```python
from build123d import *

# Parameters (mm, degrees)
SKETCH_1_W          = 8
SKETCH_1_H          = 20
EXTRUDE_1_DEPTH     = 10
EXTRUDE_1_2_DEPTH   = 10
SKETCH_2_W          = 39
SKETCH_2_H          = 15
EXTRUDE_2_DEPTH     = 2.5
CHAMFER_1_SIZE      = 1
SKETCH_3_R          = 2
CUT_EXTRUDE_1_DEPTH = 10
CUT_EXTRUDE_3_DEPTH = 10
SKETCH_6_W          = 5
SKETCH_6_H          = 17.5
EXTRUDE_3_DEPTH     = 8
SKETCH_7_W          = 5
SKETCH_7_H          = 17.5
EXTRUDE_4_DEPTH     = 8
EXTRUDE_5_REACH     = 41.825
SKETCH_8_W          = 5
SKETCH_8_H          = 11


with BuildPart() as part:
    # Sketch 1 → Extrude 1 (new body)
    with BuildSketch(Plane.XY):
        with Locations((4, 10)):
            Rectangle(SKETCH_1_W, SKETCH_1_H)
    extrude(amount=EXTRUDE_1_DEPTH)



with BuildPart() as body_2:
    # Sketch 1 → Extrude 1 2 (new body)
    with BuildSketch(Plane.XY):
        with Locations((35, 10)):
            Rectangle(SKETCH_1_W, SKETCH_1_H)
    extrude(amount=EXTRUDE_1_2_DEPTH)


with BuildPart() as part_1:
    add(part.part)

    add(body_2.part)  # Extrude 2 merges body 2
    # Sketch 2 → Extrude 2 (add)
    with BuildSketch(Plane.XZ):
        with Locations((19.5, 7.5)):
            Rectangle(SKETCH_2_W, SKETCH_2_H)
    extrude(amount=-EXTRUDE_2_DEPTH)

    # Chamfer 1
    chamfer_1_edges = [part_1.edges().sort_by_distance(p)[0] for p in [
        (19.5, 2.5, 0),
    ]]
    chamfer(chamfer_1_edges, length=CHAMFER_1_SIZE)

    # Sketch 3 → Cut-Extrude 1 (cut)
    with BuildSketch(Plane(origin=(0, 0, 0), x_dir=(-1, 0, 0), z_dir=(0, 0, -1))):
        with Locations((-35.5, 17)):
            Circle(SKETCH_3_R)
        with Locations((-3.5, 17)):
            Circle(SKETCH_3_R)
        with Locations((-35.5, 4)):
            Circle(SKETCH_3_R)
        with Locations((-3.5, 4)):
            Circle(SKETCH_3_R)
    extrude(amount=-CUT_EXTRUDE_1_DEPTH, mode=Mode.SUBTRACT)

    # Sketch 5 → Cut-Extrude 3 (cut)
    with BuildSketch(Plane(origin=(0, 2.5, 0), x_dir=(1, 0, 0), z_dir=(0, 1, 0))):
        with BuildLine():
            Line((10.4, -12), (10.4, -10))
            ThreePointArc((10.4, -10), (12, -8.4), (13.6, -10))
            Line((13.6, -10), (13.6, -12))
            ThreePointArc((13.6, -12), (12, -13.6), (10.4, -12))
        make_face()
        with BuildLine():
            Line((25.4, -12), (25.4, -10))
            ThreePointArc((25.4, -10), (27, -8.4), (28.6, -10))
            Line((28.6, -10), (28.6, -12))
            ThreePointArc((28.6, -12), (27, -13.6), (25.4, -12))
        make_face()
    extrude(amount=-CUT_EXTRUDE_3_DEPTH, mode=Mode.SUBTRACT)

    # Sketch 6 → Extrude 3 (add)
    with BuildSketch(Plane(origin=(39, 0, 0), x_dir=(0, 0, -1), z_dir=(1, 0, 0))):
        with Locations((-12.5, 11.25)):
            Rectangle(SKETCH_6_W, SKETCH_6_H)
    extrude(amount=-EXTRUDE_3_DEPTH)

    # Sketch 7 → Extrude 4 (add)
    with BuildSketch(Plane.ZY):
        with Locations((12.5, 11.25)):
            Rectangle(SKETCH_7_W, SKETCH_7_H)
    extrude(amount=-EXTRUDE_4_DEPTH)

    # Sketch 8 → Extrude 5 (add, up to next)
    with BuildSketch(Plane.ZY.offset(-31), mode=Mode.PRIVATE) as extrude_5_sk1:
        with Locations((5, 8)):
            Rectangle(SKETCH_8_W, SKETCH_8_H)
    extrude_5_tool1 = extrude(extrude_5_sk1.sketch, amount=EXTRUDE_5_REACH, mode=Mode.PRIVATE) - part_1.part
    add(extrude_5_tool1.solids().sort_by_distance((31, 8, 5))[0])


solid = part_1.part
```
Source: CAD feature listing. Evaluate the final solid. Frame: model axes, mm. A direction names the side the tool comes from. Round coordinates to 2 decimals unless told otherwise and drop trailing zeros. Loops run counter-clockwise (first coordinate to the right, second up) from the corner with the lowest first, then second, coordinate; pieces in that order, holes last.
(1) Contact query for flat-ended pins moving along their axis: pin 1 Ø1.5 at (x, z) = (21.5, 12) entering from +Y; pin 2 Ø5 at (x, y) = (24.5, 6) entering from +Z; pin 3 Ø4 at (x, z) = (20, 6) entering from +Y. Output: stop coordinate, or through.
From the geometry:
pin 1: stops at y = 2.5
pin 2: stops at z = 7.5
pin 3: stops at y = 13.5
(2) Section query C-C (z = 8). Output: boundary loops of the cut face in (x, y), and give its area (3 significant figures).
From the geometry:
outline: (0, 0) - (39, 0) - (39, 20) - (31, 20) - (31, 2.5) - (8, 2.5) - (8, 20) - (0, 20) - close; hole circle Ø4 at (3.5, 4); hole circle Ø4 at (3.5, 17); hole circle Ø4 at (35.5, 4); hole circle Ø4 at (35.5, 17)
area: 327 mm2
(3) Section query B-B (y = 17). Output: boundary loops of the cut face in (x, z).
From the geometry:
outline: (0, 0) - (1.5, 0) - (1.5, 10) - (5.5, 10) - (5.5, 0) - (8, 0) - (8, 15) - (0, 15) - close; (31, 0) - (33.5, 0) - (33.5, 10) - (37.5, 10) - (37.5, 0) - (39, 0) - (39, 15) - (31, 15) - close
(4) Section query A-A (x = 12). Output: boundary loops of the cut face in (y, z).
From the geometry:
outline: (0, 0) - (1.5, 0) - (2.5, 1) - (2.5, 2.5) - (13.5, 2.5) - (13.5, 7.5) - (2.5, 7.5) - (2.5, 8.4) - (0, 8.4) - close; (0, 13.6) - (2.5, 13.6) - (2.5, 15) - (0, 15) - close
(5) Section query D-D (x = 35.5). Output: boundary loops of the cut face in (y, z).
From the geometry:
outline: (0, 0) - (2, 0) - (2, 10) - (6, 10) - (6, 0) - (15, 0) - (15, 10) - (19, 10) - (19, 0) - (20, 0) - (20, 15) - (0, 15) - close
(6) Material intervals for probe 1 along Y at (x, z) = (3.5, 8); probe 2 along X at (y, z) = (14.5, 11.5); probe 3 along X at (y, z) = (16, 8.25), sorted ascending.
From the geometry:
probe 1: y = 0 to 2, 6 to 15, 19 to 20
probe 2: x = 0 to 8, 31 to 39
probe 3: x = 0 to 1.77, 5.23 to 8, 31 to 33.77, 37.23 to 39
(7) Pull-direction query (Y, two-part tool) for faces 1 (the cylindrical face through (27, 1.3, 13.6)), 2 (the flat face through (4, 20, 7)), 3 (the cylindrical face through (3.76, 18.983, 4.93)); classes: +Y half, -Y half, draft (parallel to the pull), parting line (faces both ways), or undercut.
From the geometry:
face 1: draft
face 2: +Y half
face 3: undercut
(8) Access query for faces 4 (the flat face through (19.3, 2, 0.5)), 5 (the flat face through (8, 13, 9)), 6 (the flat face through (3, 4, 10)), 7 (the cylindrical face through (12, 1.3, 13.6)). Directions: +Z, -Z, +X, -X, +Y, -Y. A direction counts if a zero-diameter tool reaches every point of the face in a straight line with its end or side. Return the directions, or none.
From the geometry:
face 4: -Z, +Y
face 5: +Y
face 6: -Z
face 7: +Y, -Y
